Autodesk Inventor part; units mm, degrees
ref_plane "YZ Plane" through (0, 0, 0) normal (1, 0, 0) x (0, 1, 0)
ref_plane "XZ Plane" through (0, 0, 0) normal (0, 1, 0) x (-1, 0, 0)
ref_plane "XY Plane" through (0, 0, 0) normal (0, 0, 1) x (1, 0, 0)
sketch "Sketch1" plane through (0, 0, 0) normal (0, 1, 0) x (-1, 0, 0)
  line L0 (85, 100) -> (-85, 100)
  line L1 (-85, 100) -> (-85, -100)
  line L2 (-85, -100) -> (85, -100)
  line L3 (85, -100) -> (85, 100)
  point P0 (0, 0)
  point P1 (0, -100)
  dimension "d0" = 200
  dimension "d1" = 170
  dimension "d15" = 100
  dimension "d16" = 0
extrude "Extrusion1" add sketch "Sketch1" along normal blind 4
sketch "Sketch2" plane through (85, 0, -100) normal (0, 0, -1) x (-1, 0, 0)
  line L0 (0, 4) -> (169.1447, 65.5636)
  line L1 (0, 4) -> (-1.7101, 8.6985)
  line L2 (-1.7101, 8.6985) -> (167.4346, 70.2621)
  line L3 (167.4346, 70.2621) -> (169.1447, 65.5636)
  line L4 (0, 4) -> (-10.9899, 0)
  line L5 (0, 0) -> (170, 0)
  line L6 (-10.9899, 0) -> (-12.7, 4.6985)
  line L7 (-12.7, 4.6985) -> (-1.7101, 8.6985)
  point P0 (85, 0)
  dimension "d4" = 180
  dimension "d5" = 5
  dimension "d6" = 20
  dimension "d7" = 20
extrude "Extrusion2" [suppressed]
sketch "Sketch3" plane through (0, 0, 0) normal (0, -1, 0) x (1, 0, 0)
  line L0 (-85, -100) -> (-85, 100)
  line L1 (-85, 77.5) -> (-65, 77.5)
  line L2 (-65, 77.5) -> (-65, 2.5)
  line L3 (-65, 2.5) -> (-85, 2.5)
  line L4 (-85, 2.5) -> (-85, 77.5)
  point P0 (0, 0)
  point P1 (-65, 40)
  dimension "d10" = 20
  dimension "d11" = 75
  dimension "d12" = 40
extrude "Extrusion3" cut sketch "Sketch3" against normal through all
mirror "Mirror1" about plane through (0, 0, 0) normal (1, 0, 0) of "Extrusion3"
sketch "Sketch4" plane through (0, 4, 0) normal (0, 1, 0) x (1, 0, 0)
  line L0 (25, 100) -> (-25, 100)
  line L1 (-25, 100) -> (-25, 96)
  line L2 (-25, 96) -> (25, 96)
  line L3 (25, 96) -> (25, 100)
  point P0 (0, 0)
  point P1 (0, 96)
  dimension "d17" = 4
  dimension "d18" = 96
  dimension "d19" = 50
extrude "Extrusion4" cut sketch "Sketch4" against normal through all
sketch "Sketch5" plane through (0, 4, 0) normal (0, 1, 0) x (1, 0, 0)
  line L0 (-85, 100) -> (-85, -2.5)
  line L1 (-85, 80) -> (-81, 80)
  line L2 (-81, 80) -> (-81, 30)
  line L3 (-81, 30) -> (-85, 30)
  line L4 (-85, 30) -> (-85, 80)
  line L5 (-85, -100) -> (85, -100)
  point P0 (0, 0)
  dimension "d22" = 50
  dimension "d23" = 4
  dimension "d24" = 20
extrude "Extrusion5" cut sketch "Sketch5" against normal through all
mirror "Mirror2" about plane through (0, 0, 0) normal (1, 0, 0) of "Extrusion5"
sketch "Sketch6" plane through (-85, 0, 100) normal (0, 0, 1) x (1, 0, 0)
  line L0 (150, 4) -> (170, 4)
  line L1 (0, 0) -> (170, 0)
  line L2 (170, 0) -> (170, 4)
  line L3 (170, 4) -> (0, 4)
  line L4 (0, 4) -> (0, 0)
  point P0 (85, 0)
extrude "Extrusion6" add sketch "Sketch6" along normal blind 53.169
sketch "Sketch7" plane through (0, 4, 0) normal (0, 1, 0) x (1, 0, 0)
  line L0 (-85, -77.5) -> (-85, -153.169)
  line L1 (-85, -102.5) -> (-81, -102.5)
  line L2 (-81, -102.5) -> (-81, -132.5)
  line L3 (-81, -132.5) -> (-85, -132.5)
  line L4 (-85, -132.5) -> (-85, -102.5)
  line L5 (-65, -77.5) -> (-85, -77.5)
  point P0 (0, 0)
  point P1 (-83, -102.5)
  dimension "d32" = 30
  dimension "d33" = 4
  dimension "d34" = 25
extrude "Extrusion7" cut sketch "Sketch7" against normal blind 10
mirror "Mirror3" about plane through (0, 0, 0) normal (1, 0, 0) of "Extrusion7"
properties part number "Parte inf"
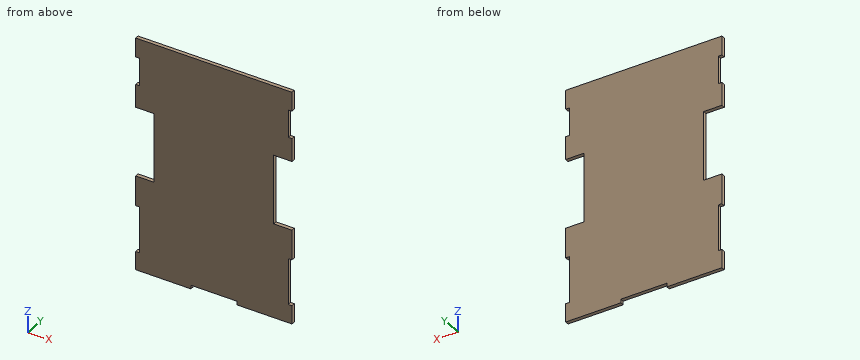
Read the model definition and answer for the solid it produces. Units are mm, in the model's axes. Round coordinates to 2 decimals unless told otherwise and drop trailing zeros. Write each loop counter-clockwise with the first axis right and the second up, starting at its lowest first coordinate (ties: lowest second). Pieces come first, ordered by that corner, then holes.
Q1. Flat-ended cylindrical pins translate along their axes: P1, Ø2, axis at y = 2.5, z = 47.5, coming from the +X side; P2, Ø1.2, axis at y = 1.5, z = 111.5, coming from the +X side; P3, Ø2, axis at y = 1, z = 36.5, coming from the -X side. Find the tip coordinate at first contact, or state that the pin passes through.
Values:
P1: stops at x = 65
P2: stops at x = 81
P3: stops at x = -65
Q2. Find section C-C on x = 21.5. Determine the outline of the cut face in (y, z).
Values:
outline: (0, -96) - (4, -96) - (4, 153.17) - (0, 153.17) - close
Q3. Straight lines are drawn through the part: line 1 (Z direction, x = -67.5, y = 0.2); line 2 (Z direction, x = -10.5, y = 0.35); line 3 (X direction, y = 1.6, z = 51.5). For each, find the intervals that lie inside material, in ascending order.
Values:
line 1: z = -100 to 2.5, 77.5 to 153.17
line 2: z = -96 to 153.17
line 3: x = -65 to 65
Q4. Find section B-B on z = 30.5. Determine the outline of the cut face in (x, y).
Values:
outline: (-65, 0) - (65, 0) - (65, 4) - (-65, 4) - close
